Autodesk Inventor part; units mm, degrees
ref_plane "YZ Plane" through (0, 0, 0) normal (1, 0, 0) x (0, 1, 0)
ref_plane "XZ Plane" through (0, 0, 0) normal (0, 1, 0) x (-1, 0, 0)
ref_plane "XY Plane" through (0, 0, 0) normal (0, 0, 1) x (1, 0, 0)
sketch "Sketch1" plane through (0, 0, 0) normal (0, 0, 1) x (1, 0, 0)
  line L0 (14.4828, 12.3536) -> (49.4828, 12.3536)
  line L1 (49.4828, 12.3536) -> (49.4828, 27.3536)
  line L2 (14.4828, 12.3536) -> (14.4828, 27.3536)
  line L3 (54.4828, 27.3536) -> (54.4828, 7.3536)
  line L4 (54.4828, 7.3536) -> (9.4828, 7.3536)
  line L5 (9.4828, 7.3536) -> (9.4828, 27.3536)
  line L6 (9.4828, 27.3536) -> (14.4828, 27.3536)
  line L7 (49.4828, 27.3536) -> (54.4828, 27.3536)
  point P0 (0, 0)
  dimension "d0" = 35
  dimension "d1" = 15
  dimension "d2" = 15
  dimension "d3" = 5
extrude "Extrusion1" add sketch "Sketch1" along normal blind 70
sketch "Sketch3" plane through (54.4828, 7.3536, 0) normal (1, 0, 0) x (0, 0, -1)
  line L0 (0, 20) -> (0, 0)
  line L1 (0, 5) -> (-70, 5)
  line L2 (0, 20) -> (-25, 20)
  line L3 (-25, 20) -> (-25, 5)
  line L4 (-25, 5) -> (0, 5)
  line L5 (0, 5) -> (0, 20)
  point P0 (0, -7.3536)
  dimension "d6" = 25
extrude "Extrusion2" cut sketch "Sketch3" against normal blind 5
properties part number "outlifting"
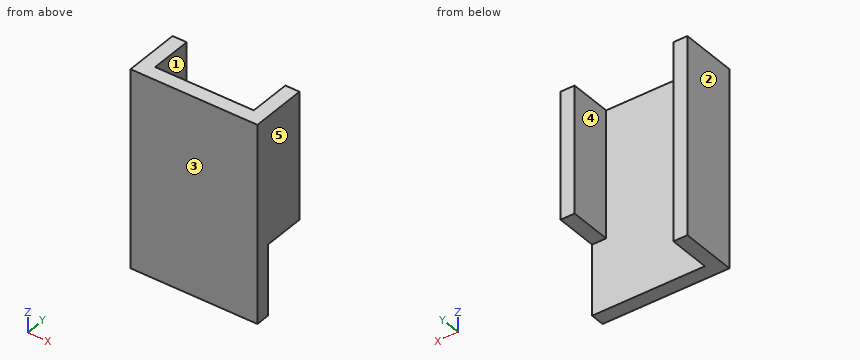
Work out the finished part from the listing and answer in its coordinate system (mm). Face numbers are marked on the shaded views. A direction names the side the tool comes from. Coordinates: 2 decimals unless noted, no trailing zeros. Loops run counter-clockwise (first coordinate to the right, second up) from the corner with the lowest first, then second, coordinate; pieces in that order, holes last. Notation, with made-up numbers: (-30, 56) -> (8, 56) arc R24 cw to (8, 89) -> close; hole circle Ø3 at (-3.5, 68). An arc over 180 degrees is marked (long way). Answer as CSV lines item,"result".
Q1. Each of these flat-tipped pins is pushed along its axis until it touches: pin 1 (5 mm diameter, centred on x = 25.5, z = 34.5, fed in from +Y); pin 2 (1.5 mm diameter, centred on x = 53, y = 23, fed in from -Z). Where does it stop, or does it pass through?
Findings:
pin 1,"stops at y = 12.35"
pin 2,"stops at z = 25"
Q2. Find the intervals of material crossed by probe 1 along Y at (x, z) = (44, 30); probe 2 along X at (y, z) = (15, 40); probe 3 along Z at (x, y) = (50, 23.5), in increasing order.
Findings:
probe 1,"y = 7.35 to 12.35"
probe 2,"x = 9.48 to 14.48, 49.48 to 54.48"
probe 3,"z = 25 to 70"
Q3. The part is cut by section A-A on y = 14. Write down the section's boundary in (x, z).
Findings:
outline,"(9.48, 0) -> (14.48, 0) -> (14.48, 70) -> (9.48, 70) -> close; (49.48, 25) -> (54.48, 25) -> (54.48, 70) -> (49.48, 70) -> close"
Q4. The part is cut by section D-D on z = 20.5. Write down the section's boundary in (x, y), and give its area (3 significant figures).
Findings:
outline,"(9.48, 7.35) -> (54.48, 7.35) -> (54.48, 12.35) -> (14.48, 12.35) -> (14.48, 27.35) -> (9.48, 27.35) -> close"
area,"300 mm²"
Q5. The part is cut by section C-C on x = 15.5. Write down the section's boundary in (y, z).
Findings:
outline,"(7.35, 0) -> (12.35, 0) -> (12.35, 70) -> (7.35, 70) -> close"
Q6. The part is cut by section B-B on z = 40. Write down the section's boundary in (x, y), and give its area (3 significant figures).
Findings:
outline,"(9.48, 7.35) -> (54.48, 7.35) -> (54.48, 27.35) -> (49.48, 27.35) -> (49.48, 12.35) -> (14.48, 12.35) -> (14.48, 27.35) -> (9.48, 27.35) -> close"
area,"375 mm²"
Q7. A tool of negligible diameter and unlimited length cuts with its end or side. For the marked faces 4 and 5, from which of +Z, -Z, +X, -X, +Y, -Y can it reach the whole face along a straight path? Write none if from no direction.
Findings:
face 4,"+Z, -Z, +Y"
face 5,"+Z, -Z, +X, +Y, -Y"
Q8. For a pull along X with two mould halves and no side action, classify the marked faces 1, 2 and 3 as +X half, -X half, draft (parallel to the pull), parting line (faces both ways), or undercut.
Findings:
face 1,"undercut"
face 2,"-X half"
face 3,"draft"
